Design review of the part built by this model. Coordinates are the model's own, in mm. Give positions to 0.01 mm unless a question says otherwise; leave off trailing zeros. Loops run counter-clockwise (first coordinate to the right, second up) from the corner with the lowest first, then second, coordinate; pieces in that order, holes last. Notation, with made-up numbers: M 4,-4.5 L 9,-4.5 A25 cw 9,16.5 Z; hole C 30.5,39.25 d1. An arc over 180 degrees is marked long. Use CSV: the item, a comma, the result in double quotes.
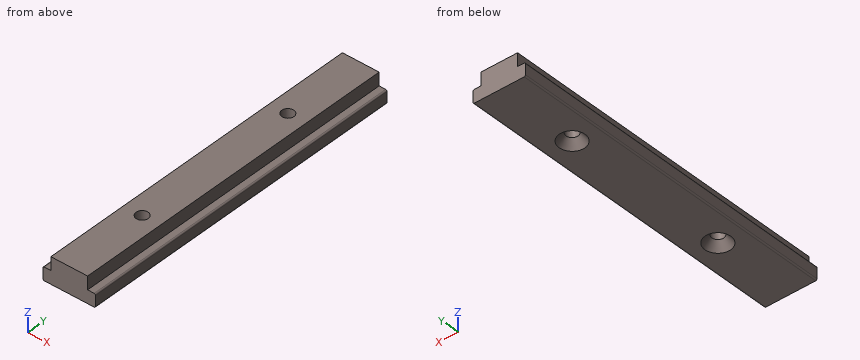
from build123d import *

# Parameters (mm, degrees)
F1_DEPTH       = 101.6
F3_R           = 0.396875
F4_D           = 3.6576
F4_CSINK_D     = 7.7978
F4_CSINK_ANGLE = 82


with BuildPart() as f1:
    # F0 (on Front) → F1 (new body)
    with BuildSketch(Plane.XZ):
        Polygon((0, 3.96875), (0, 0), (15.875, 0), (15.875, 3.96875), (13.49375, 3.96875), (13.49375, 7.9375), (2.38125, 7.9375), (2.38125, 3.96875), align=None)
    extrude(amount=F1_DEPTH)

    # F3
    f3_edges = [f1.edges().sort_by_distance(p)[0] for p in [
        (15.875, -50.8, 3.96875),
        (15.875, -50.8, 0),
        (0, -50.8, 3.96875),
        (0, -50.8, 0),
    ]]
    fillet(f3_edges, radius=F3_R)

    # F4 (through all)
    with Locations(Plane(origin=(0, 0, 0), x_dir=(1, 0, 0), z_dir=(0, 0, -1))):
        with Locations((7.9375, 76.2), (7.9375, 25.4)):
            CounterSinkHole(F4_D / 2, F4_CSINK_D / 2, counter_sink_angle=F4_CSINK_ANGLE)


solid = f1.part
(1) We need section B-B on z = 6.5. State the section outline as (x, y) points, then the cut area to 3 significant figures.
A:
outline,"M 2.38,-101.6 L 13.49,-101.6 L 13.49,0 L 2.38,0 Z; hole C 7.94,-76.2 d3.66; hole C 7.94,-25.4 d3.66"
area,"1,110 mm²"
(2) We need section C-C on y = -65.5. State the section outline as (x, z) points (1 decimal), then the cut area to 3 significant figures.
A:
outline,"M 0,0.4 A0.4 ccw 0.4,0 L 15.5,0 A0.4 ccw 15.9,0.4 L 15.9,3.6 A0.4 ccw 15.5,4 L 13.5,4 L 13.5,7.9 L 2.4,7.9 L 2.4,4 L 0.4,4 A0.4 ccw 0,3.6 Z"
area,"107 mm²"
(3) We need section A-A on y = -25.4. State the section outline as (x, z) points (1 decimal), then the cut area to 3 significant figures.
A:
outline,"M 0,0.4 A0.4 ccw 0.4,0 L 4,0 L 6.1,2.4 L 6.1,7.9 L 2.4,7.9 L 2.4,4 L 0.4,4 A0.4 ccw 0,3.6 Z; M 9.8,2.4 L 11.8,0 L 15.5,0 A0.4 ccw 15.9,0.4 L 15.9,3.6 A0.4 ccw 15.5,4 L 13.5,4 L 13.5,7.9 L 9.8,7.9 Z"
area,"73.0 mm²"
(4) Clearance check with flat-ended pins moving along their axes: P1, Ø2, axis at x = 11.5, z = 4, coming from the +Y side; P2, Ø1, axis at y = -48.5, z = 6, coming from the -X side; P3, Ø1.6, axis at x = 1.5, y = -51, coming from the +Z side; P4, Ø2, axis at x = 7.94, y = -76.2, coming from the -Z side. State where each tip first meets the part, or that it passes through.
A:
P1,"y = 0"
P2,"x = 2.38"
P3,"z = 3.97"
P4,"through"
(5) Wall thickness on line 1 along Y through (x, z) = (8, 6.75); line 2 along X through (y, z) = (-76.2, 5.55); line 3 along Y through (x, z) = (5.25, 1): over which ranges is each line inside the solid? List them lowest first. Write a range as [from, to].
A:
line 1,"[-101.6, -78.03], [-74.37, -27.23], [-23.57, 0]"
line 2,"[2.38, 6.11], [9.77, 13.49]"
line 3,"[-101.6, -77.6], [-74.8, -26.8], [-24, 0]"
